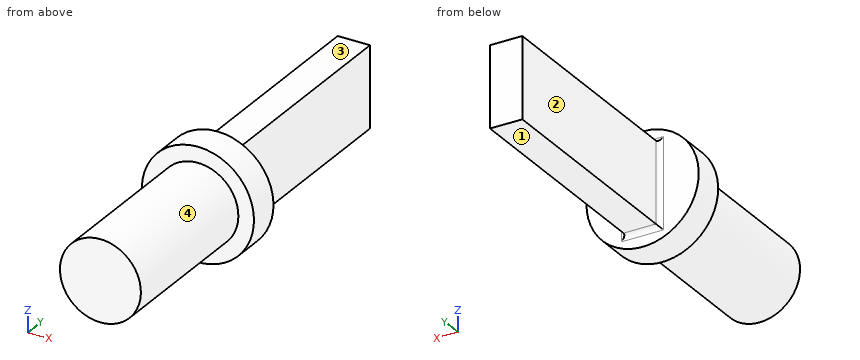
from build123d import *

# Parameters (mm, degrees)
SKETCH1_R           = 17.325
BOSS_EXTRUDE1_DEPTH = 10
SKETCH2_R           = 12.5
BOSS_EXTRUDE2_DEPTH = 50
SKETCH3_W           = 10
SKETCH3_H           = 25
BOSS_EXTRUDE3_DEPTH = 70
FILLET1_R           = 1.5


with BuildPart() as part:
    # Sketch1 → Boss-Extrude1 (new body)
    with BuildSketch(Plane(origin=(0, 0, 0), x_dir=(1, 0, 0), z_dir=(0, 1, 0))):
        with Locations(Location((0, 0, 0), (0, 0, 270))):
            Circle(SKETCH1_R)
    extrude(amount=-BOSS_EXTRUDE1_DEPTH)

    # Sketch2 → Boss-Extrude2 (add)
    with BuildSketch(Plane.XZ.offset(10)):
        with Locations(Location((0, 0, 0), (0, 0, 270))):
            Circle(SKETCH2_R)
    extrude(amount=BOSS_EXTRUDE2_DEPTH)

    # Sketch3 → Boss-Extrude3 (add)
    with BuildSketch(Plane(origin=(0, 0, 0), x_dir=(1, 0, 0), z_dir=(0, 1, 0))):
        Rectangle(SKETCH3_W, SKETCH3_H)
    extrude(amount=BOSS_EXTRUDE3_DEPTH)

    # Fillet1
    fillet1_edges = [part.edges().sort_by_distance(p)[0] for p in [
        (5, 0, 0),
        (0, 0, -12.5),
        (-5, 0, 0),
        (0, 0, 12.5),
    ]]
    fillet(fillet1_edges, radius=FILLET1_R)


solid = part.part
Geometry check sheet. Reference: the model listing, model coordinates, mm. Face numbers are marked on the shaded views. A direction names the side the tool comes from. Give positions to 0.01 mm unless a question says otherwise; leave off trailing zeros. Loops run counter-clockwise (first coordinate to the right, second up) from the corner with the lowest first, then second, coordinate; pieces in that order, holes last. Notation, with made-up numbers: M 79.5,77 L 129.5,77 A28 ccw 129.5,97 Z; hole C -37.5,37 d1. An arc over 180 degrees is marked long. Answer as a JSON object with one key per item and string values. Group by question number.
Item 1: Sectioned sample at D-D on y = 24. Record the boundary of the cut face in (x, z).
Item 2: Sectioned sample at A-A on x = 0. Record the boundary of the cut face in (y, z) (3 decimals).
Item 3: Gauge pin test, flat ends, axial feed: pin 1 (4 mm diameter, centred on x = 0, y = -21, fed in from +Z); pin 2 (1.5 mm diameter, centred on x = -7.5, z = 4.5, fed in from +Y); pin 3 (3 mm diameter, centred on y = 25.5, z = 8, fed in from -X). Record the tip position at first contact, or that the pin passes through.
Item 4: Access from +Z, -Z, +X, -X, +Y, -Y to the whole of each face (thin tool, end or side, straight path). Record for the marked faces 1, 2, 3 and 4.
Item 5: Material ranges on L1, parallel to Z at x = -2.5, y = 5.5; L2, parallel to Y at x = 15, z = 1.5; L3, parallel to X at y = 49.5, z = -2.5, recorded low to high.
Item 6: Sectioned sample at C-C on y = -11.5. Record the boundary of the cut face in (x, z), plus the area to 3 significant figures.
Item 7: Sectioned sample at B-B on z = 0. Record the boundary of the cut face in (x, y) (3 decimals).
Findings below:
{
 "1": {"outline": "M -5,-12.5 L 5,-12.5 L 5,12.5 L -5,12.5 Z"},
 "2": {"outline": "M -60,-12.5 L -10,-12.5 L -10,-17.325 L 0,-17.325 L 0,-14 A1.5 cw 1.5,-12.5 L 70,-12.5 L 70,12.5 L 1.5,12.5 A1.5 cw 0,14 L 0,17.325 L -10,17.325 L -10,12.5 L -60,12.5 Z"},
 "3": {"pin 1": "z = 12.5", "pin 2": "y = 0", "pin 3": "x = -5"},
 "4": {"face 1": "-Z, +X, -X, +Y", "face 2": "+Z, -Z, -X, +Y", "face 3": "+Z, +X, -X, +Y", "face 4": "-Y"},
 "5": {"L1": "-12.5 to 12.5", "L2": "-10 to 0", "L3": "-5 to 5"},
 "6": {"outline": "C 0,0 d25", "area": "491 mm2"},
 "7": {"outline": "M -17.325,-10 L -12.5,-10 L -12.5,-60 L 12.5,-60 L 12.5,-10 L 17.325,-10 L 17.325,0 L 6.5,0 A1.5 cw 5,1.5 L 5,70 L -5,70 L -5,1.5 A1.5 cw -6.5,0 L -17.325,0 Z"}
}
